Autodesk Inventor part; units mm, degrees
ref_plane "Work Plane1" through (0, 0, 0) normal (1, 0, 0) x (0, 1, 0)
ref_plane "XZ Plane" through (0, 0, 0) normal (0, 1, 0) x (-1, 0, 0)
ref_plane "XY Plane" through (0, 0, 0) normal (0, 0, 1) x (1, 0, 0)
sketch "Sketch1" plane through (0, 0, 0) normal (0, 0, 1) x (1, 0, 0)
  circle A0 centre (0, 0) radius 10.2
  dimension "d0" = 20.4
extrude "Extrusion1" add sketch "Sketch1" along normal blind 25.1
ref_plane "Work Plane1" through (0, 0, 0) normal (1, 0, 0) x (0, 1, 0)
sketch "Sketch2" plane through (0, 0, 0) normal (1, 0, 0) x (0, 1, 0)
  line L0 (10.2, 25.1) -> (-10.2, 25.1)
  line L1 (10.2, 25.1) -> (-10.2, 25.1)
  line L2 (-10.2, 25.1) -> (-10.2, 0)
  line L3 (-10.2, 0) -> (10.2, 0)
  line L4 (10.2, 0) -> (10.2, 25.1)
  line L5 (0, 0) -> (7.7, 0)
  line L6 (7.7, 0) -> (7.7, 25.1)
  line L7 (7.7, 25.1) -> (0, 25.1)
  line L8 (0, 25.1) -> (0, 0)
  line L9 (10.2, 0) -> (-10.2, 0)
  line L10 (7.7, 25.1) -> (10.2, 25.1)
  line L11 (10.2, 25.1) -> (10.2, 0)
  line L12 (10.2, 0) -> (7.7, 0)
  line L13 (7.7, 0) -> (7.7, 25.1)
  line L14 (0, 25.1) -> (-7.7, 25.1)
  line L15 (-7.7, 25.1) -> (-7.7, 0)
  line L16 (-7.7, 0) -> (0, 0)
  line L17 (0, 0) -> (0, 25.1)
  line L18 (-7.7, 0) -> (-10.2, 0)
  line L19 (-10.2, 0) -> (-10.2, 25.1)
  line L20 (-10.2, 25.1) -> (-7.7, 25.1)
  line L21 (-7.7, 25.1) -> (-7.7, 0)
  dimension "d4" = 7.7
  dimension "d5" = 7.7
extrude "Extrusion2" cut sketch "Sketch2" along normal mid plane 22 contours L4 L3 L6 L0 | L15 L3 L2 L0
sketch "Sketch3" plane through (0, 0, 25.1) normal (0, 0, 1) x (1, 0, 0)
  circle A0 centre (0, 0) radius 3.075
  circle A1 centre (0, 0) radius 1
  dimension "d8" = 6.15
  dimension "d9" = 2
extrude "Extrusion3" add sketch "Sketch3" along normal blind 1.6
sketch "Sketch4" plane through (-6.6895, 7.7, 25.1) normal (0, 1, 0) x (1, 0, 0)
  line L0 (0, 0) -> (0, 25.1)
  line L1 (13.3791, 25.1) -> (13.3791, 0)
  line L2 (0, 25.1) -> (13.3791, 25.1)
  line L3 (13.3791, 25.1) -> (13.3791, 21.6)
  line L4 (13.3791, 21.6) -> (0, 21.6)
  line L5 (0, 21.6) -> (0, 25.1)
  point P0 (6.6895, 25.1)
  dimension "d12" = 3.5
extrude "Extrusion4" add sketch "Sketch4" along normal blind 0.8
sketch "Sketch5" plane through (0, 0, 0) normal (0, 0, -1) x (-1, 0, 0)
  circle A0 centre (0, 0) radius 4.75
  line L0 (-3.5382, -3.1691) -> (3.5382, -3.1691)
  dimension "d15" = 9.5
extrude "Extrusion6" add sketch "Sketch5" along normal blind 1.6 contours A0 L0 picked at (0.1876, -0.5406)
properties part number "DCMotor"
Input: part model. Units: mm. Frame: model coordinates. A direction names the side the tool comes from. Give positions to 0.01 mm unless a question says otherwise; leave off trailing zeros. Write each loop counter-clockwise with the first axis right and the second up, starting at its lowest first coordinate (ties: lowest second). Pieces come first, ordered by that corner, then holes.
Q1. Material intervals for probe 1 along Y at (x, z) = (0, 25.6) (3 decimals); probe 2 along Z at (x, y) = (-5.25, -1); probe 3 along Y at (x, z) = (-6, 8.5), sorted ascending.
Q2. Set-up query: faces 4 (the face through (0, 0, 25.1)), 5 (the face through (0, -3.169, -1)), 6 (the face through (0.153, 4.748, -0.789)), 7 (the face through (0, 7.7, 12)). Return all of +Z, -Z, +X, -X, +Y, -Y with unobstructed straight access to the full face (end or side cutting, diameter ignored); none if empty.
Q3. First-contact query: P1, Ø5, axis at y = 5.5, z = 22, coming from the -X side; P2, Ø1.3, axis at x = -1.5, z = -0.5, coming from the -Y side; P3, Ø6.5, axis at x = 0.5, z = 9, coming from the +Y side; P4, Ø3, axis at x = 7, y = -3, coming from the -Z side. Flat tips, straight axial feed; report the tip coordinate or a pass-through.
Q4. Pull-direction query (Y, two-part tool) for faces 1 (the face through (-10.2, -0.1, 12.4)), 2 (the face through (0, 4, 25.1)), 3 (the face through (0, 1, 26)); classes: pulls with the +Y half, pulls with the -Y half, needs draft (parallel to the pull), parting line crosses it, or undercut.
Q5. Section D-D, the plane y = 1.75. Output: boundary loops of the cut face in (x, z).
Q6. Section A-A, the plane x = 0. Output: boundary loops of the cut face in (y, z) (3 decimals), plus the area to 3 significant figures.
Q7. Section B-B, the plane y = 0. Output: boundary loops of the cut face in (x, z) (3 decimals), plus the area to 3 significant figures.
Q8. Section C-C, the plane z = 19.5. Output: boundary loops of the cut face in (x, y), plus the area to 3 significant figures.
Filled in:
1. probe 1: y = -3.075 to -1, 1 to 3.075
1. probe 2: z = 0 to 25.1
1. probe 3: y = -7.7 to 7.7
2. face 4: +Z
2. face 5: -Z, +X, -X, -Y
2. face 6: -Z
2. face 7: +Z, +X, -X, +Y
3. P1: stops at x = -9.75
3. P2: stops at y = -7.7
3. P3: stops at y = 7.7
3. P4: stops at z = 0
4. face 1: parting line crosses it
4. face 2: needs draft
4. face 3: undercut
5. outline: (-10.05, 0) - (-4.42, 0) - (-4.42, -1.6) - (4.42, -1.6) - (4.42, 0) - (10.05, 0) - (10.05, 25.1) - (2.53, 25.1) - (2.53, 26.7) - (-2.53, 26.7) - (-2.53, 25.1) - (-10.05, 25.1) - close
6. outline: (-7.7, 0) - (-3.169, 0) - (-3.169, -1.6) - (4.75, -1.6) - (4.75, 0) - (8.5, 0) - (8.5, 3.5) - (7.7, 3.5) - (7.7, 25.1) - (3.075, 25.1) - (3.075, 26.7) - (1, 26.7) - (1, 25.1) - (-1, 25.1) - (-1, 26.7) - (-3.075, 26.7) - (-3.075, 25.1) - (-7.7, 25.1) - close
6. area: 409 mm2
7. outline: (-10.2, 0) - (-4.75, 0) - (-4.75, -1.6) - (4.75, -1.6) - (4.75, 0) - (10.2, 0) - (10.2, 25.1) - (3.075, 25.1) - (3.075, 26.7) - (1, 26.7) - (1, 25.1) - (-1, 25.1) - (-1, 26.7) - (-3.075, 26.7) - (-3.075, 25.1) - (-10.2, 25.1) - close
7. area: 534 mm2
8. outline: (-6.69, -7.7) - (6.69, -7.7) arc R10.2 ccw to (6.69, 7.7) - (-6.69, 7.7) arc R10.2 ccw to start
8. area: 281 mm2
